from build123d import *

# Parameters (mm, degrees)
SKETCH1_R           = 20
SKETCH1_R_2         = 1.5
SKETCH1_R_3         = 2
SKETCH1_R_4         = 1.4
BOSS_EXTRUDE1_DEPTH = 3.2


with BuildPart() as part:
    # Sketch1 → Boss-Extrude1 (new body)
    with BuildSketch(Plane(origin=(0, 0, 0), x_dir=(1, 0, 0), z_dir=(0, 1, 0))):
        with BuildLine():
            Line((283, 55), (283, -55))
            ThreePointArc((283, -55), (281.535533906, -58.535533906), (278, -60))
            Line((278, -60), (133.66563146, -60))
            ThreePointArc((133.66563146, -60), (132.967201164, -60.125914857), (132.35671362, -60.487804878))
            ThreePointArc((132.35671362, -60.487804878), (0, 0), (132.35671362, 60.487804878))
            ThreePointArc((132.35671362, 60.487804878), (132.967201164, 60.125914857), (133.66563146, 60))
            Line((133.66563146, 60), (278, 60))
            ThreePointArc((278, 60), (281.535533906, 58.535533906), (283, 55))
        make_face()
        with Locations(Location((80, 0, 0), (0, 0, 270))):
            Circle(SKETCH1_R, mode=Mode.SUBTRACT)
        with Locations(Location((7.5, 0, 0), (0, 0, 270))):
            Circle(SKETCH1_R_2, mode=Mode.SUBTRACT)
        with Locations(Location((28.734758364, 51.265241636, 0), (0, 0, 270))):
            Circle(SKETCH1_R_2, mode=Mode.SUBTRACT)
        with Locations(Location((80, 72.5, 0), (0, 0, 270))):
            Circle(SKETCH1_R_2, mode=Mode.SUBTRACT)
        with Locations(Location((131.265241636, 51.265241636, 0), (0, 0, 270))):
            Circle(SKETCH1_R_2, mode=Mode.SUBTRACT)
        with Locations(Location((131.265241636, -51.265241636, 0), (0, 0, 270))):
            Circle(SKETCH1_R_2, mode=Mode.SUBTRACT)
        with Locations(Location((80, -72.5, 0), (0, 0, 270))):
            Circle(SKETCH1_R_2, mode=Mode.SUBTRACT)
        with Locations(Location((28.734758364, -51.265241636, 0), (0, 0, 270))):
            Circle(SKETCH1_R_2, mode=Mode.SUBTRACT)
        with Locations(Location((32.5, 0, 0), (0, 0, 270))):
            Circle(SKETCH1_R_3, mode=Mode.SUBTRACT)
        with Locations(Location((80, 47.5, 0), (0, 0, 270))):
            Circle(SKETCH1_R_3, mode=Mode.SUBTRACT)
        with Locations(Location((127.5, 0, 0), (0, 0, 270))):
            Circle(SKETCH1_R_3, mode=Mode.SUBTRACT)
        with Locations(Location((80, -47.5, 0), (0, 0, 270))):
            Circle(SKETCH1_R_3, mode=Mode.SUBTRACT)
        with Locations(Location((270.75, 51, 0), (0, 0, 270))):
            Circle(SKETCH1_R_2, mode=Mode.SUBTRACT)
        with Locations(Location((270.75, -51, 0), (0, 0, 270))):
            Circle(SKETCH1_R_2, mode=Mode.SUBTRACT)
        with Locations(Location((163.5, 20, 0), (0, 0, 270))):
            Circle(SKETCH1_R_4, mode=Mode.SUBTRACT)
        with Locations(Location((163.5, -20, 0), (0, 0, 270))):
            Circle(SKETCH1_R_4, mode=Mode.SUBTRACT)
        with Locations(Location((157.75, 6.8, 0), (0, 0, 270))):
            Circle(SKETCH1_R_2, mode=Mode.SUBTRACT)
        with Locations(Location((200.75, 6.8, 0), (0, 0, 270))):
            Circle(SKETCH1_R_2, mode=Mode.SUBTRACT)
        with BuildLine():
            Line((157.5, -29), (257.5, -29))
            ThreePointArc((257.5, -29), (259, -27.5), (257.5, -26))
            Line((257.5, -26), (157.5, -26))
            ThreePointArc((157.5, -26), (156, -27.5), (157.5, -29))
        make_face(mode=Mode.SUBTRACT)
        with BuildLine():
            Line((257.5, 26), (157.5, 26))
            ThreePointArc((157.5, 26), (156, 27.5), (157.5, 29))
            Line((157.5, 29), (257.5, 29))
            ThreePointArc((257.5, 29), (259, 27.5), (257.5, 26))
        make_face(mode=Mode.SUBTRACT)
    extrude(amount=BOSS_EXTRUDE1_DEPTH)


solid = part.part
Geometry check sheet. Reference: the model listing, model coordinates, mm. Round coordinates to 2 decimals unless told otherwise and drop trailing zeros. Loops run counter-clockwise (first coordinate to the right, second up) from the corner with the lowest first, then second, coordinate; pieces in that order, holes last. Notation, with made-up numbers: (-6.75, 79) -> (43.25, 79) arc R14 cw to (43.25, 105) -> close; hole circle Ø11 at (48, -18). An arc over 180 degrees is marked (long way). Answer as a JSON object with one key per item and string values. Group by question number.
Item 1: Release check for a two-part mould opening along X. For faces 1 (the face through (281, 2, -59)), 2 (the face through (60.476, 1.578, -4.336)), 3 (the face through (143, 3.2, -1)) record: pulls with the +X half, pulls with the -X half, needs draft (parallel to the pull), parting line crosses it, or undercut.
Item 2: Cross-section at D-D, the plane x = 94. Record the cut outline in (y, z).
Item 3: Cross-section at A-A, the plane x = 178. Record the cut outline in (y, z), plus the area to 3 significant figures.
Item 4: Cross-section at C-C, the plane y = 2.4. Count the separate pieces of the cut face and the enclosed holes in it, plus the area to 3 significant figures.
Item 5: Thickness scan on line 1 along Z through (x, y) = (172.5, 1.25); line 2 along Z through (x, y) = (163.5, 1.05); line 3 along X through (y, z) = (1.65, 0). Record the ranges inside material, lowest first.
Item 6: Cross-section at B-B, the plane z = -14. Record the cut outline in (x, y), plus the area to 3 significant figures.
Item 7: Depth check by flat-ended pin: pin 1 Ø5 at (x, z) = (131.27, 51.27) entering from +Y; pin 2 Ø1.6 at (x, y) = (202, 1.5) entering from +Z. Enter the tip coordinate at first touch or a pass-through.
Determined:
{
 "1": {"face 1": "pulls with the +X half", "face 2": "undercut", "face 3": "needs draft"},
 "2": {"outline": "(0, -78.77) -> (3.2, -78.77) -> (3.2, -14.28) -> (0, -14.28) -> close; (0, 14.28) -> (3.2, 14.28) -> (3.2, 78.77) -> (0, 78.77) -> close"},
 "3": {"outline": "(0, -60) -> (3.2, -60) -> (3.2, -29) -> (0, -29) -> close; (0, -26) -> (3.2, -26) -> (3.2, 26) -> (0, 26) -> close; (0, 29) -> (3.2, 29) -> (3.2, 60) -> (0, 60) -> close", "area": "365 mm²"},
 "4": {"separate pieces": "1", "enclosed holes": "20", "area": "33,800 mm²"},
 "5": {"line 1": "z = -60 to -29, -26 to 26, 29 to 60", "line 2": "z = -60 to -29, -26 to -21.4, -18.6 to 18.6, 21.4 to 26, 29 to 60", "line 3": "x = 0 to 6, 9 to 30.5, 34.5 to 60, 100 to 125.5, 129.5 to 283"},
 "6": {"outline": "(1.23, 0) -> (65.72, 0) -> (65.72, 3.2) -> (1.23, 3.2) -> close; (94.28, 0) -> (283, 0) -> (283, 3.2) -> (94.28, 3.2) -> close", "area": "810 mm²"},
 "7": {"pin 1": "stops at y = 3.2", "pin 2": "stops at z = 60"}
}
